```python
from build123d import *

# Parameters (mm, degrees)
SKETCH1_W           = 49
SKETCH1_H           = 53
BOSS_EXTRUDE1_DEPTH = 20
SKETCH3_W           = 45
SKETCH3_H           = 49
CUT_EXTRUDE1_DEPTH  = 18
CUT_EXTRUDE2_DEPTH  = 34
CUT_EXTRUDE3_DEPTH  = 21.6
BOSS_EXTRUDE4_DEPTH = 53
BOSS_EXTRUDE5_DEPTH = 21.6
CUT_EXTRUDE4_DEPTH  = 18
CUT_EXTRUDE5_DEPTH  = 18
BOSS_EXTRUDE6_DEPTH = 18
SKETCH16_R          = 1
BOSS_EXTRUDE7_DEPTH = 18
SKETCH17_W          = 13.959273649
SKETCH17_H          = 5.98254585
CUT_EXTRUDE7_DEPTH  = 2


with BuildPart() as part:
    # Sketch1 → Boss-Extrude1 (new body)
    with BuildSketch(Plane(origin=(0, 0, 0), x_dir=(1, 0, 0), z_dir=(0, 1, 0))):
        with Locations((-6.199798715, -1.247894993)):
            Rectangle(SKETCH1_W, SKETCH1_H)
    extrude(amount=BOSS_EXTRUDE1_DEPTH)

    # Sketch3 → Cut-Extrude1 (cut)
    with BuildSketch(Plane.XZ):
        with Locations((-6.199798715, 1.247894993)):
            Rectangle(SKETCH3_W, SKETCH3_H)
    extrude(amount=-CUT_EXTRUDE1_DEPTH, mode=Mode.SUBTRACT)

    # Sketch4 → Cut-Extrude2 (cut)
    with BuildSketch(Plane.XY.offset(27.747894993)):
        Polygon((18.300201285, 20), (-3.299798715, 20), (18.300201285, 10), align=None)
    extrude(amount=-CUT_EXTRUDE2_DEPTH, mode=Mode.SUBTRACT)

    # Sketch6 → Cut-Extrude3 (cut)
    with BuildSketch(Plane(origin=(18.300201285, 0, 0), x_dir=(0, 0, -1), z_dir=(1, 0, 0))):
        Polygon((6.252105007, 10.006685103), (25.252105007, 20), (6.252105007, 20), align=None)
    extrude(amount=-CUT_EXTRUDE3_DEPTH, mode=Mode.SUBTRACT)

    # Sketch8 → Boss-Extrude4 (add)
    with BuildSketch(Plane.XY.offset(27.747894993)):
        Polygon((-1.339670196, 17.990564534), (-3.299798715, 19), (-3.299798715, 20), (-1.339670196, 19.092533093), (16.300201285, 10.925925926), (18.300201285, 10), (18.300201285, 8.793988713), (16.300201285, 9.823957367), align=None)
    extrude(amount=-BOSS_EXTRUDE4_DEPTH)

    # Sketch11 → Boss-Extrude5 (add)
    with BuildSketch(Plane(origin=(18.300201285, 0, 0), x_dir=(0, 0, -1), z_dir=(1, 0, 0))):
        Polygon((25.252105007, 20), (6.252105007, 10.006685103), (8.400320892, 10.006685103), (25.252105007, 18.870115905), align=None)
    extrude(amount=-BOSS_EXTRUDE5_DEPTH)

    # Sketch12 → Cut-Extrude4 (cut)
    with BuildSketch(Plane.XY.offset(-23.252105007)):
        Polygon((-3.299798715, 17.818188021), (-3.299798715, 10.006685103), (15.905509375, 10.006685103), (-0.967336928, 17.818188021), align=None)
    extrude(amount=CUT_EXTRUDE4_DEPTH, mode=Mode.SUBTRACT)

    # Sketch13 → Cut-Extrude5 (cut)
    with BuildSketch(Plane.ZY.offset(-16.300201285)):
        Polygon((-23.252105007, 17.818188021), (-23.252105007, 9.823957367), (-19.905888942, 9.823957367), (-8.052905944, 9.823957367), (-19.905888942, 16.058199029), align=None)
    extrude(amount=CUT_EXTRUDE5_DEPTH, mode=Mode.SUBTRACT)

    # Sketch15 → Boss-Extrude6 (add)
    with BuildSketch(Plane.XY.offset(-23.252105007)):
        Polygon((-3.299798715, 19), (-3.299798715, 18), (-1.339670196, 17.990564534), align=None)
    extrude(amount=BOSS_EXTRUDE6_DEPTH)

    # Sketch16 → Boss-Extrude7 (add)
    with BuildSketch(Plane.XZ.offset(-18)):
        with Locations((-26.249798715, 23.297894993)):
            Circle(SKETCH16_R)
        with Locations((-5.749798715, 23.297894993)):
            Circle(SKETCH16_R)
        with Locations((-26.249798715, -20.802105007)):
            Circle(SKETCH16_R)
        with Locations((-5.749798715, -20.802105007)):
            Circle(SKETCH16_R)
    extrude(amount=BOSS_EXTRUDE7_DEPTH)

    # Sketch17 → Cut-Extrude7 (cut)
    with BuildSketch(Plane(origin=(0, 0, -25.252105007), x_dir=(-1, 0, 0), z_dir=(0, 0, -1))):
        Polygon((14.456637368, 16.607010477), (12.63034375, 16.059122392), (12.63034375, 14.207010477), (20.63034375, 14.207010477), (20.63034375, 16.059122392), (18.456257111, 16.607010477), align=None)
        with Locations((-5.611259633, 11.265470537)):
            Rectangle(SKETCH17_W, SKETCH17_H)
    extrude(amount=-CUT_EXTRUDE7_DEPTH, mode=Mode.SUBTRACT)


solid = part.part
```
Work out the finished part from the listing and answer in its coordinate system (mm). A direction names the side the tool comes from. Round coordinates to 2 decimals unless told otherwise and drop trailing zeros. Write each loop counter-clockwise with the first axis right and the second up, starting at its lowest first coordinate (ties: lowest second). Pieces come first, ordered by that corner, then holes.
1) A cutting plane is placed at D-D on x = -10. Determine the outline of the cut face in (y, z), and give its area (3 significant figures).
2) Flat-ended cylindrical pins translate along their axes: P1, Ø2, axis at x = -2.5, z = 12.5, coming from the -Y side; P2, Ø1, axis at x = 4, z = -7.5, coming from the -Y side; P3, Ø0.6, axis at x = 7.5, z = -24.5, coming from the +Y side; P4, Ø0.6, axis at x = -16.5, z = -24, coming from the -Y side. Find the tip coordinate at first contact, or state that the pin passes through.
3) Determine the mould class of faces 1 (the face through (10.051, 16.044, -17.73)), 2 (the face through (-1.368, 11, -24)), 3 (the face through (16.3, 5, 1)) for opening direction Z: pulls with the +Z half, pulls with the -Z half, needs draft (parallel to the pull), parting line crosses it, or undercut.
4) Which of the six approach directions +Z, -Z, +X, -X, +Y, -Y give full straight-line access (tool end or side, diameter ignored) to faces 4 (the face through (-26, 0, 23)), 5 (the face through (-7, 9, -23.252)), 6 (the face through (-12.63, 15, -24))?
5) Consider probe 1 along Z at (x, y) = (9, 8); probe 2 along X at (y, z) = (2.75, -2.5); probe 3 along X at (y, z) = (5, 23.5). Determine where each line is inside the solid, lowest interval first.
6) A cutting plane is placed at A-A on y = 2.25. Determine the outline of the cut face in (x, z), and give its area (3 significant figures).
7) A cutting plane is placed at B-B on x = 7.5. Determine the outline of the cut face in (y, z), and give its area (3 significant figures).
Entries:
1. outline: (0, -25.25) - (20, -25.25) - (20, 27.75) - (0, 27.75) - (0, 25.75) - (18, 25.75) - (18, -23.25) - (0, -23.25) - close
1. area: 178 mm2
2. P1: stops at y = 18
2. P2: stops at y = 15.29
2. P3: stops at y = 19.76
2. P4: stops at y = 0
3. face 1: pulls with the +Z half
3. face 2: needs draft
3. face 3: undercut
4. face 4: +Z, -Z, +X, -X, -Y
4. face 5: -Y
4. face 6: -Z
5. probe 1: z = -25.25 to -23.25, 25.75 to 27.75
5. probe 2: x = -30.7 to -28.7, 16.3 to 18.3
5. probe 3: x = -30.7 to -28.7, -27.23 to -25.27, -6.73 to -4.77, 16.3 to 18.3
6. outline: (-30.7, -25.25) - (18.3, -25.25) - (18.3, 27.75) - (-30.7, 27.75) - close; circle Ø2 at (-26.25, -20.8); circle Ø2 at (-26.25, 23.3); circle Ø2 at (-5.75, -20.8); circle Ø2 at (-5.75, 23.3); hole (-28.7, -23.25) - (16.3, -23.25) - (16.3, 25.75) - (-28.7, 25.75) - close
6. area: 405 mm2
7. outline: (0, -25.25) - (8.27, -25.25) - (8.27, -23.25) - (0, -23.25) - close; (0, 25.75) - (13.9, 25.75) - (13.9, -15.8) - (17.82, -23.25) - (14.26, -23.25) - (14.26, -25.25) - (20, -25.25) - (15, -15.75) - (15, 27.75) - (0, 27.75) - close
7. area: 111 mm2
